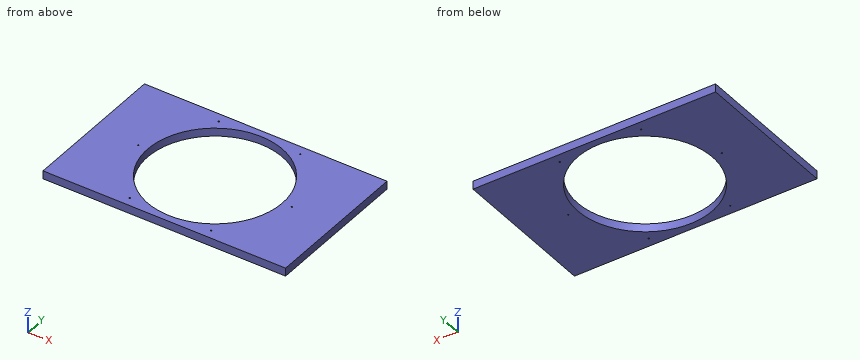
```python
from build123d import *

# Parameters (mm, degrees)
SKETCH1_W           = 180
SKETCH1_H           = 110
BOSS_EXTRUDE1_DEPTH = 6
SKETCH2_R           = 50
CUT_EXTRUDE1_DEPTH  = 6
SKETCH4_R           = 0.5
CUT_EXTRUDE2_DEPTH  = 40


with BuildPart() as part:
    # Sketch1 → Boss-Extrude1 (new body)
    with BuildSketch(Plane.XY):
        with Locations((90, 55)):
            Rectangle(SKETCH1_W, SKETCH1_H)
    extrude(amount=BOSS_EXTRUDE1_DEPTH)

    # Sketch2 → Cut-Extrude1 (cut)
    with BuildSketch(Plane.XY):
        with Locations((90, 55)):
            Circle(SKETCH2_R)
    extrude(amount=CUT_EXTRUDE1_DEPTH, mode=Mode.SUBTRACT)

    # Sketch4 → Cut-Extrude2 (cut)
    with BuildSketch(Plane.XY):
        with Locations((59.794601939, 103.338741481)):
            Circle(SKETCH4_R)
        with Locations((120.205398061, 103.338741481)):
            Circle(SKETCH4_R)
        with Locations((147, 55)):
            Circle(SKETCH4_R)
        with Locations((120.205398061, 6.661258519)):
            Circle(SKETCH4_R)
        with Locations((59.794601939, 6.661258519)):
            Circle(SKETCH4_R)
        with Locations((33, 55)):
            Circle(SKETCH4_R)
    extrude(amount=CUT_EXTRUDE2_DEPTH, mode=Mode.SUBTRACT)


solid = part.part
```
Work out the finished part from the listing and answer in its coordinate system (mm). Round coordinates to 2 decimals unless told otherwise and drop trailing zeros. Loops run counter-clockwise (first coordinate to the right, second up) from the corner with the lowest first, then second, coordinate; pieces in that order, holes last. Notation, with made-up numbers: (18.25, -38.5) -> (54.25, -38.5) arc R21 ccw to (54.25, -2.5) -> close; hole circle Ø3 at (75, -8). An arc over 180 degrees is marked (long way). Write each question's results on one line, items separated by ' | '. Start each with the question number.
1. Find the intervals of material crossed by probe 1 along Y at (x, z) = (147, 4.75); probe 2 along Y at (x, z) = (90, 3.65); probe 3 along X at (y, z) = (84, 5.15), in increasing order. Write a range as from..to.
2. Section B-B (y = 87) is taken. Determine the outline of the cut face in (x, z), plus the area to 3 significant figures.
3. Section C-C (z = 1.3) is taken. Determine the outline of the cut face in (x, y), plus the area to 3 significant figures.
4. Section A-A (x = 90) is taken. Determine the outline of the cut face in (y, z), plus the area to 3 significant figures.
Evaluation:
1) probe 1: y = 0..54.5, 55.5..110 | probe 2: y = 0..5, 105..110 | probe 3: x = 0..49.27, 130.73..180
2) outline: (0, 0) -> (51.58, 0) -> (51.58, 6) -> (0, 6) -> close; (128.42, 0) -> (180, 0) -> (180, 6) -> (128.42, 6) -> close | area: 619 mm2
3) outline: (0, 0) -> (180, 0) -> (180, 110) -> (0, 110) -> close; hole circle Ø1 at (33, 55); hole circle Ø100 at (90, 55); hole circle Ø1 at (59.79, 6.66); hole circle Ø1 at (59.79, 103.34); hole circle Ø1 at (120.21, 6.66); hole circle Ø1 at (120.21, 103.34); hole circle Ø1 at (147, 55) | area: 11,900 mm2
4) outline: (0, 0) -> (5, 0) -> (5, 6) -> (0, 6) -> close; (105, 0) -> (110, 0) -> (110, 6) -> (105, 6) -> close | area: 60.0 mm2
